Input: part model. Units: mm. Frame: model coordinates. A direction names the side the tool comes from. Coordinates: 2 decimals unless noted, no trailing zeros. Order: outer loops, then holes, each group sorted by start corner. A loop starts at its lowest first (then second) coordinate and runs counter-clockwise, first axis right, second up. Notation, with made-up numbers: (22, -38.5) -> (60, -38.5) arc R21 cw to (60, -5.5) -> close; hole circle Ø3 at (46, -36.5). An arc over 180 degrees is marked (long way). One line per item, written item: value. Start each with the question number.
from build123d import *

# Parameters (mm, degrees)
SKETCH_01_W                   = 70
SKETCH_01_H                   = 56
EXTRUDE_01_DEPTH              = 6
SKETCH_02_W                   = 70
SKETCH_02_H                   = 46
EXTRUDE_02_DEPTH              = 6
EXTRUDE_03_DEPTH              = 4
EXTRUDE_START                 = 66
EXTRUDE_04_DEPTH              = 4
CUT_EXTRUDE_05_4_3_DEPTH      = 99.163129534
CUT_EXTRUDE_05_4_3_DEPTH_BACK = 99.163129534
SKETCH_05_R                   = 11.25
SKETCH_05_R_2                 = 1.7
CUT_EXTRUDE_06_DEPTH          = 99.163129534
CUT_EXTRUDE_06_DEPTH_BACK     = 99.163129534
CUT_EXTRUDE_07_4_4_DEPTH      = 99.163129534
CUT_EXTRUDE_07_4_4_DEPTH_BACK = 99.163129534
SKETCH_07_R                   = 2.25


with BuildPart() as part:
    # 01_Пластина_эскиз → 01_Передняя_пластина (new body)
    with BuildSketch(Plane.XY):
        with Locations((35, 28)):
            Rectangle(SKETCH_01_W, SKETCH_01_H)
    extrude(amount=EXTRUDE_01_DEPTH)

    # 02_Полка_эскиз → 02_Полка (add)
    with BuildSketch(Plane(origin=(0, 0, 0), x_dir=(1, 0, 0), z_dir=(0, 1, 0))):
        with Locations((35, 17)):
            Rectangle(SKETCH_02_W, SKETCH_02_H)
    extrude(amount=EXTRUDE_02_DEPTH)

    # 03_Косынка_левая_эскиз → 03_Косынка_левая (add)
    with BuildSketch(Plane(origin=(0, 0, 0), x_dir=(0, 0, -1), z_dir=(1, 0, 0))):
        Polygon((40, 6), (0, 6), (0, 36), align=None)
    extrude(amount=EXTRUDE_03_DEPTH)

    # 04_Косынка_правая_эскиз → 04_Косынка_правая (add)
    with BuildSketch(Plane(origin=(0, 0, 0), x_dir=(0, 0, -1), z_dir=(1, 0, 0)).offset(EXTRUDE_START)):
        Polygon((40, 6), (0, 6), (0, 36), align=None)
    extrude(amount=EXTRUDE_04_DEPTH)

    # 05_Мотор_передний_фланец_эскиз → 05_Буртик_и_4_отверстия_М3 (cut, two sides: drawn at the far end of the back side and taken through both)
    with BuildSketch(Plane.XY.offset(-CUT_EXTRUDE_05_4_3_DEPTH_BACK)):
        with Locations((35, 27.15)):
            Circle(SKETCH_05_R)
        with Locations((19.5, 11.65)):
            Circle(SKETCH_05_R_2)
        with Locations((19.5, 42.65)):
            Circle(SKETCH_05_R_2)
        with Locations((50.5, 11.65)):
            Circle(SKETCH_05_R_2)
        with Locations((50.5, 42.65)):
            Circle(SKETCH_05_R_2)
    extrude(amount=CUT_EXTRUDE_05_4_3_DEPTH + CUT_EXTRUDE_05_4_3_DEPTH_BACK, mode=Mode.SUBTRACT)

    # 06_Свод_45град_эскиз → 06_Свод_отверстия_для_печати (cut, two sides: drawn at the far end of the back side and taken through both)
    with BuildSketch(Plane.XY.offset(-CUT_EXTRUDE_06_DEPTH_BACK)):
        Polygon((27.045048712, 35.104951288), (42.954951288, 35.104951288), (35, 43.059902577), align=None)
    extrude(amount=CUT_EXTRUDE_06_DEPTH + CUT_EXTRUDE_06_DEPTH_BACK, mode=Mode.SUBTRACT)

    # 07_Крепление_полки_эскиз → 07_4_отверстия_М4 (cut, two sides: drawn at the far end of the back side and taken through both)
    with BuildSketch(Plane(origin=(0, 0, 0), x_dir=(1, 0, 0), z_dir=(0, 1, 0)).offset(-CUT_EXTRUDE_07_4_4_DEPTH_BACK)):
        with Locations(Location((8.5, 12, 0), (0, 0, 270))):
            Circle(SKETCH_07_R)
        with Locations(Location((8.5, 30, 0), (0, 0, 270))):
            Circle(SKETCH_07_R)
        with Locations(Location((61.5, 12, 0), (0, 0, 270))):
            Circle(SKETCH_07_R)
        with Locations(Location((61.5, 30, 0), (0, 0, 270))):
            Circle(SKETCH_07_R)
    extrude(amount=CUT_EXTRUDE_07_4_4_DEPTH + CUT_EXTRUDE_07_4_4_DEPTH_BACK, mode=Mode.SUBTRACT)


solid = part.part
1) Section query D-D, the plane z = -12. Return the cut outline in (x, y).
2) Mould query, pull axis Y, two halves, no side actions, for faces 1 (the flat face through (27, 16, 6)), 2 (the flat face through (35, 56, 3)), 3 (the cylindrical face through (19.279, 44.336, 2.958)). Classes: +Y half, -Y half, draft (parallel to the pull), parting line (faces both ways), or undercut.
3) Section query A-A, the plane x = 61.5. Return the cut outline in (y, z), plus the area to 3 significant figures.
4) Access query for faces 4 (the flat face through (31.08, 39.14, 2.96)), 5 (the flat face through (35, 6, -20)), 6 (the flat face through (70, 16, -12)). Directions: +Z, -Z, +X, -X, +Y, -Y. A direction counts if a zero-diameter tool reaches every point of the face in a straight line with its end or side. Return the directions, or none.
5) Section query B-B, the plane y = 27.15. Return the cut outline in (x, z), plus the area to 3 significant figures.
6) Pin query (flat end, axial travel): pin 1 Ø5.5 at (x, y) = (50.5, 42.65) entering from -Z; pin 2 Ø5 at (y, z) = (7.5, -21.5) entering from -X; pin 3 Ø5 at (x, z) = (8.5, -30) entering from +Y. Return the tip coordinate at first contact, or that it passes through.
7) Section query C-C, the plane z = 1.5. Return the cut outline in (x, y).
8) Ray query, line 1 along Y through (x, z) = (19.5, 3.15); line 2 along Z through (x, y) = (8.5, 3.35); line 3 along X through (y, z) = (1.4, -12). Return the intervals inside material, ascending. Write a range as from..to.
Entries:
1. outline: (0, 0) -> (6.25, 0) -> (6.25, 6) -> (4, 6) -> (4, 27) -> (0, 27) -> close; (10.75, 0) -> (59.25, 0) -> (59.25, 6) -> (10.75, 6) -> close; (63.75, 0) -> (70, 0) -> (70, 27) -> (66, 27) -> (66, 6) -> (63.75, 6) -> close
2. face 1: draft
2. face 2: +Y half
2. face 3: undercut
3. outline: (0, -40) -> (6, -40) -> (6, -32.25) -> (0, -32.25) -> close; (0, -27.75) -> (6, -27.75) -> (6, -14.25) -> (0, -14.25) -> close; (0, -9.75) -> (6, -9.75) -> (6, 0) -> (56, 0) -> (56, 6) -> (0, 6) -> close
3. area: 522 mm2
4. face 4: +Z, -Z
4. face 5: -Z, +Y
4. face 6: +Z, -Z, +X, +Y, -Y
5. outline: (0, -11.8) -> (4, -11.8) -> (4, 0) -> (23.75, 0) -> (23.75, 6) -> (0, 6) -> close; (46.25, 0) -> (66, 0) -> (66, -11.8) -> (70, -11.8) -> (70, 6) -> (46.25, 6) -> close
5. area: 379 mm2
6. pin 1: stops at z = 0
6. pin 2: stops at x = 0
6. pin 3: stops at y = 6
7. outline: (0, 0) -> (70, 0) -> (70, 56) -> (0, 56) -> close; hole circle Ø3.4 at (19.5, 11.65); hole circle Ø3.4 at (19.5, 42.65); hole (27.05, 35.1) arc R11.25 ccw (long way) to (42.95, 35.1) -> (35, 43.06) -> close; hole circle Ø3.4 at (50.5, 11.65); hole circle Ø3.4 at (50.5, 42.65)
8. line 1: y = 0..9.95, 13.35..40.95, 44.35..56
8. line 2: z = -40..-32.25, -27.75..-14.25, -9.75..6
8. line 3: x = 0..6.25, 10.75..59.25, 63.75..70
